from build123d import *

# Parameters (mm, degrees)
F0_W      = 609.6
F0_H      = 609.6
F1_DEPTH  = 3.175
F2_W      = 457.2
F2_H      = 304.8
F2_W_2    = 3.175
F2_H_2    = 152.4
F2_W_3    = 76.2
F2_H_3    = 3.175
F2_H_4    = 6.35
F3_DEPTH  = 3.176
F4_W      = 3.175
F4_H      = 101.6
F5_DEPTH  = 3.176
F6_W      = 3.175
F6_H      = 203.2
F7_DEPTH  = 3.176
F8_W      = 25.4
F8_H      = 3.175
F9_DEPTH  = 25.4
F10_W     = 3.175
F10_H     = 114.3
F11_DEPTH = 3.175


with BuildPart() as f1:
    # F0 (on Front) → F1 (new body)
    with BuildSketch(Plane.XZ):
        Rectangle(F0_W, F0_H)
    extrude(amount=F1_DEPTH)

    # F2 (on face) → F3 (cut, through all)
    with BuildSketch(Plane.XZ.offset(3.175)):
        with Locations((-0.080462, -152.4)):
            Rectangle(F2_W, F2_H)
        with Locations((-277.892962, 228.6)):
            Rectangle(F2_W_2, F2_H_2)
        with Locations((277.732038, 228.6)):
            Rectangle(F2_W_2, F2_H_2)
        Polygon((283.913076, 54.01643), (304.719538, 68.585271), (304.719538, 72.461231), (282.091971, 56.617238), align=None)
        with Locations((-190.580462, 36.5125)):
            Rectangle(F2_W_3, F2_H_3)
        with Locations((-0.080462, 36.5125)):
            Rectangle(F2_W_3, F2_H_3)
        with Locations((190.419538, 36.5125)):
            Rectangle(F2_W_3, F2_H_3)
        with Locations((-190.580462, 301.625)):
            Rectangle(F2_W_3, F2_H_4)
        with Locations((190.419538, 301.625)):
            Rectangle(F2_W_3, F2_H_4)
    extrude(amount=-F3_DEPTH, mode=Mode.SUBTRACT)

    # F4 (on face) → F5 (cut, through all)
    with BuildSketch(Plane(origin=(0, 0, 0), x_dir=(-1, 0, 0), z_dir=(0, 1, 0))):
        with Locations((-277.8125, -254)):
            Rectangle(F4_W, F4_H)
        with Locations((277.8125, -254)):
            Rectangle(F4_W, F4_H)
    extrude(amount=-F5_DEPTH, mode=Mode.SUBTRACT)

    # F6 (on face) → F7 (cut, through all)
    with BuildSketch(Plane(origin=(0, 0, 0), x_dir=(-1, 0, 0), z_dir=(0, 1, 0))):
        with Locations((284.242962, 152.4)):
            Rectangle(F6_W, F6_H)
    extrude(amount=-F7_DEPTH, mode=Mode.SUBTRACT)

    # F8 (on face) → F9 (cut)
    with BuildSketch(Plane.XZ.offset(3.175)):
        with Locations((0, 33.3375)):
            Rectangle(F8_W, F8_H)
    extrude(amount=-F9_DEPTH, mode=Mode.SUBTRACT)

    # F10 (on face) → F11 (join)
    with BuildSketch(Plane.XZ.offset(3.175)):
        with Locations((-277.892962, 209.55)):
            Rectangle(F10_W, F10_H)
        with Locations((277.732038, 209.55)):
            Rectangle(F10_W, F10_H)
    extrude(amount=-F11_DEPTH)


solid = f1.part
Build history of the part. All positions in model axes, mm. Give positions to 0.01 mm unless a question says otherwise; leave off trailing zeros. Order: outer loops, then holes, each group sorted by start corner. A loop starts at its lowest first (then second) coordinate and runs counter-clockwise, first axis right, second up. Notation, with made-up numbers: M -22.5,-15 L -10.5,-15 A25 cw -10.5,5 Z; hole C 43,-13 d5. An arc over 180 degrees is marked long. Use one line per item in the form item = value.
1) Drop flat-ended pins along their axis: pin 1 (1 mm diameter, centred on x = -277.5, y = -1, fed in from +Z); pin 2 (1 mm diameter, centred on x = -206, y = -1.5, fed in from +Z); pin 3 (1 mm diameter, centred on x = -74, y = -2.5, fed in from -Z). Give the stop position or say it passes through.
Calculated:
pin_1 = 266.7
pin_2 = 298.45
pin_3 = 0
2) Saw through at A-A (x = -179). Give the cut face in (y, z) (3 decimals), plus the area to 4 significant figures.
Calculated:
outline = M -3.175,0 L 0,0 L 0,34.925 L -3.175,34.925 Z; M -3.175,38.1 L 0,38.1 L 0,298.45 L -3.175,298.45 Z
area = 937.5 mm2
3) Saw through at C-C (y = -1.3). State how many separate pieces and enclosed holes the cut face has, plus the area to 3 significant figures.
Calculated:
separate_pieces = 1
enclosed_holes = 5
area = 229,000 mm2
4) Saw through at B-B (z = -75). Give the cut face in (x, y) (3 decimals), plus the area to 3 significant figures.
Calculated:
outline = M -304.8,-3.175 L -228.68,-3.175 L -228.68,0 L -304.8,0 Z; M 228.52,-3.175 L 304.8,-3.175 L 304.8,0 L 228.52,0 Z
area = 484 mm2
5) Probe probe 1 along X at (y, z) = (-2.75, 104); probe 2 along X at (y, z) = (-0.4, 271); probe 3 along X at (y, z) = (-0.5, -123). List the from-to ranges inside material, lowest first.
Calculated:
probe_1 = -304.8 to -285.83, -282.66 to 304.8
probe_2 = -304.8 to -279.48, -276.31 to 276.14, 279.32 to 304.8
probe_3 = -304.8 to -228.68, 228.52 to 304.8
6) Two-plate mould, pull along Z, no slides. Class faces 1 (the face through (-4, -3.175, 72)), 2 (the face through (294.17, -1.61, 61.2)): released by +Z, released by -Z, zero draft, split by the parting line, or undercut.
Calculated:
face_1 = zero draft
face_2 = undercut
